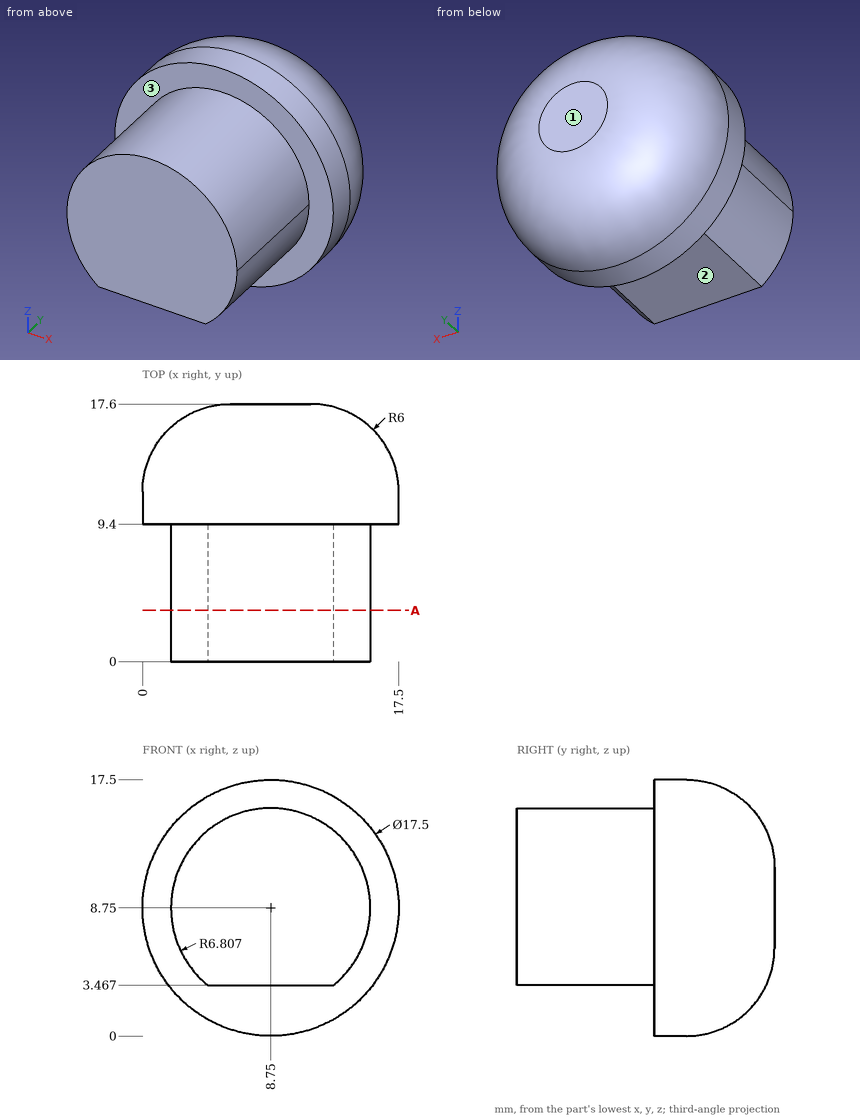
The figure shows three views and two pictorial views of one solid part (mm, origin at its lowest corner). Answer the questions. A direction names the side the tool comes from. Round coordinates to 2 decimals unless told otherwise and drop trailing zeros. Write each loop counter-clockwise with the first axis right and the second up, starting at its lowest first coordinate (ties: lowest second). Pieces come first, ordered by that corner, then holes. Notation, with made-up numbers: M 19,18.5 L 47,18.5 A34 cw 47,57.5 Z; hole C 87.5,36 d7. An arc over 180 degrees is marked long. Write each question's results on one line, items separated by ' | '. Start each with the question number.
(1) Each of these flat-tipped pins is pushed along its axis until it touches: P1, Ø5, axis at y = 10.5, z = 2.5, coming from the +X side; P2, Ø2, axis at x = 14.5, y = 10, coming from the -Z side; P3, Ø8, axis at x = 4, y = 11.5, coming from the +Z side. Where does it stop, or does it pass through?
(2) For the marked faces 1, 2 and 3, determine the directions among +Z, -Z, +X, -X, +Y, -Y from which every point of the face is accessible in a straight line to the end or side of a thin tool.
(3) Find the intervals of material crossed by line 1 (X direction, y = 15.75, z = 4.75) (1 decimal); line 2 (Z direction, x = 3, y = 5); line 3 (Z direction, x = 10, y = 14.5) (1 decimal), in increasing order.
(4) The part is cut by section A-A, the plane y = 3.5. Write down the section's boundary in (x, z), and give its area (3 significant figures).
Worked answers:
1) P1: stops at x = 16.66 | P2: stops at z = 1.4 | P3: stops at z = 17.47
2) face 1: +Z, -Z, +X, -X, +Y | face 2: -Z, +X, -X, -Y | face 3: -Y
3) line 1: x = 2.9 to 14.6 | line 2: z = 5.11 to 12.39 | line 3: z = 0.8 to 16.7
4) outline: M 4.46,3.47 L 13.04,3.47 A6.81 ccw long Z | area: 137 mm²
